The listing builds one solid part. Answer for the finished solid, in the listing's coordinates (mm). Coordinates: 2 decimals unless noted, no trailing zeros. Loops run counter-clockwise (first coordinate to the right, second up) from the corner with the lowest first, then second, coordinate; pieces in that order, holes last. Notation, with made-up numbers: M -4.75,60.25 L 15.25,60.25 A15 cw 15.25,86.25 Z; hole C 56.5,-36.5 d7. An arc over 180 degrees is marked long. Answer as a JSON object with one key per item and string values. Group by question number.
1. A cutting plane is placed at A-A on y = -18.5. Give the vertices of the cut face in (x, z) (3 decimals).
2. Determine the mould class of faces 1 (the face through (57.15, -13, 9)), 2 (the face through (3.62, -12.88, 34.28)), 3 (the face through (41.4, -12.88, 23.52)), 4 (the face through (22, 0, 19)) for opening direction X: released by +X, released by -X, zero draft, split by the parting line, or undercut.
3. A cutting plane is placed at C-C on x = 8. Give the vertices of the cut face in (y, z).
4. Straight lines are drawn through the part: L1, parallel to Z at x = 12.5, y = -10.25; L2, parallel to X at y = -11, z = 29; L3, parallel to X at y = -14, z = 21.5. For each, find the intervals that lie inside material, in ascending order.
5. A cutting plane is placed at B-B on z = 34. Give the vertices of the cut face in (x, y).
6. Given pin 1 (1 mm diameter, centred on y = -15.5, z = 32, fed in from -X); pin 2 (5 mm diameter, centred on x = 9, y = -22, fed in from +Z), each flat-ended and moving along its own axis, determine where each tip first touches the part or whether it passes through.
from build123d import *

# Parameters (mm, degrees)
F0_W     = 57.15
F0_H     = 38.1
F1_DEPTH = 25.4
F2_R     = 12.7
F4_DEPTH = 25.4


with BuildPart() as f1:
    # F0 (on Front) → F1 (new body)
    with BuildSketch(Plane.XZ):
        with Locations((28.575, 19.05)):
            Rectangle(F0_W, F0_H)
    extrude(amount=F1_DEPTH)

    # F2
    f2_edges = [f1.edges().sort_by_distance(p)[0] for p in [
        (0, -12.7, 38.1),
    ]]
    fillet(f2_edges, radius=F2_R)

    # F3 (on face) → F4 (cut)
    with BuildSketch(Plane.XZ.offset(25.4)):
        with BuildLine():
            Line((57.15, 38.1), (34.925, 38.1))
            ThreePointArc((34.925, 38.1), (41.575556, 23.369399), (57.15, 19.05))
            Line((57.15, 19.05), (57.15, 38.1))
        make_face()
    extrude(amount=-F4_DEPTH, mode=Mode.SUBTRACT)


solid = f1.part
From the geometry:
{
 "1": {"outline": "M 0,0 L 57.15,0 L 57.15,19.05 A19.05 cw 34.925,38.1 L 12.7,38.1 A12.7 ccw 0,25.4 Z"},
 "2": {"face 1": "released by +X", "face 2": "released by -X", "face 3": "undercut", "face 4": "zero draft"},
 "3": {"outline": "M -25.4,0 L 0,0 L 0,37.2 L -25.4,37.2 Z"},
 "4": {"L1": "z = 0 to 38.1", "L2": "x = 0.52 to 37.09", "L3": "x = 0 to 44.17"},
 "5": {"outline": "M 3.35,-25.4 L 35.31,-25.4 L 35.31,0 L 3.35,0 Z"},
 "6": {"pin 1": "stops at x = 1.56", "pin 2": "stops at z = 38.04"}
}
